Can you work these out from the model? Positions are in its coordinate system, mm. Round coordinates to 2 decimals unless told otherwise and drop trailing zeros. Order: outer loops, then holes, each group sorted by start corner. A loop starts at its lowest first (then second) coordinate and runs counter-clockwise, first axis right, second up. Notation, with made-up numbers: (-19, 85.25) -> (-10, 85.25) arc R10 ccw to (-10, 96.25) -> close; hole circle Ø2 at (72.5, -16). An arc over 180 degrees is marked (long way). Use a Markdown table: item, result. Add a question column.
Q1. We'd pull the mould along Z, two halves only. Please class faces 1 (the face through (0, 5, 125)), 2 (the face through (0.187, 4.93, 93.254)), 3 (the face through (25, 5, 51)): +Z half, -Z half, draft (parallel to the pull), parting line (faces both ways), or undercut.
Q2. If we section it at C-C on x = -12: List the corners of the cut face in (y, z) for me.
Q3. I need wall thicknesses on line 1 along X through (y, z) = (7.5, 97.5); line 2 along X through (y, z) = (6.5, 0); line 3 along Z through (x, y) = (1.5, 9). Which ranges of each line are inside material? Lowest first, please. Write a range as [from, to].
Q4. If we section it at B-B on z = 0: List the corners of the cut face in (x, y) for me, plus the area to 3 significant figures.
Q5. If we section it at A-A on x = 0: List the corners of the cut face in (y, z) for me.
Q6. I'm going to push a flat-ended pin straight in: pin 1 Ø10 at (x, z) = (0, 111.5) entering from -Y. Where does the tip first touch, or does it pass through?
Q7. If we section it at D-D on y = 6.5: List the corners of the cut face in (x, z) for me, plus the area to 3 significant figures.
```python
from build123d import *

# Parameters (mm, degrees)
SKETCH1_W           = 50
SKETCH1_H           = 150
SKETCH1_R           = 15
BOSS_EXTRUDE1_DEPTH = 10
SKETCH2_R           = 4.25
CUT_EXTRUDE1_DEPTH  = 10


with BuildPart() as part:
    # Sketch1 → Boss-Extrude1 (new body)
    with BuildSketch(Plane(origin=(0, 0, 0), x_dir=(1, 0, 0), z_dir=(0, 1, 0))):
        with Locations((0, -50)):
            Rectangle(SKETCH1_W, SKETCH1_H)
        with Locations(Location((0, 0, 0), (0, 0, 270))):
            Circle(SKETCH1_R, mode=Mode.SUBTRACT)
    extrude(amount=BOSS_EXTRUDE1_DEPTH)

    # Sketch2 → Cut-Extrude1 (cut)
    with BuildSketch(Plane(origin=(0, 0, 0), x_dir=(1, 0, 0), z_dir=(0, 1, 0))):
        with Locations(Location((0, -111.5, 0), (0, 0, 270))):
            Circle(SKETCH2_R)
        with Locations(Location((0, -97.5, 0), (0, 0, 270))):
            Circle(SKETCH2_R)
    extrude(amount=CUT_EXTRUDE1_DEPTH, mode=Mode.SUBTRACT)


solid = part.part
```
Answer below:
| question | item | result |
|---|---|---|
| 1 | face 1 | +Z half |
| 1 | face 2 | undercut |
| 1 | face 3 | draft |
| 2 | outline | (0, -25) -> (10, -25) -> (10, -9) -> (0, -9) -> close; (0, 9) -> (10, 9) -> (10, 125) -> (0, 125) -> close |
| 3 | line 1 | [-25, -4.25], [4.25, 25] |
| 3 | line 2 | [-25, -15], [15, 25] |
| 3 | line 3 | [-25, -14.92], [14.92, 93.52], [101.48, 107.52], [115.48, 125] |
| 4 | outline | (-25, 0) -> (-15, 0) -> (-15, 10) -> (-25, 10) -> close; (15, 0) -> (25, 0) -> (25, 10) -> (15, 10) -> close |
| 4 | area | 200 mm² |
| 5 | outline | (0, -25) -> (10, -25) -> (10, -15) -> (0, -15) -> close; (0, 15) -> (10, 15) -> (10, 93.25) -> (0, 93.25) -> close; (0, 101.75) -> (10, 101.75) -> (10, 107.25) -> (0, 107.25) -> close; (0, 115.75) -> (10, 115.75) -> (10, 125) -> (0, 125) -> close |
| 6 | pin 1 | y = 0 |
| 7 | outline | (-25, -25) -> (25, -25) -> (25, 125) -> (-25, 125) -> close; hole circle Ø30 at (0, 0); hole circle Ø8.5 at (0, 97.5); hole circle Ø8.5 at (0, 111.5) |
| 7 | area | 6,680 mm² |
